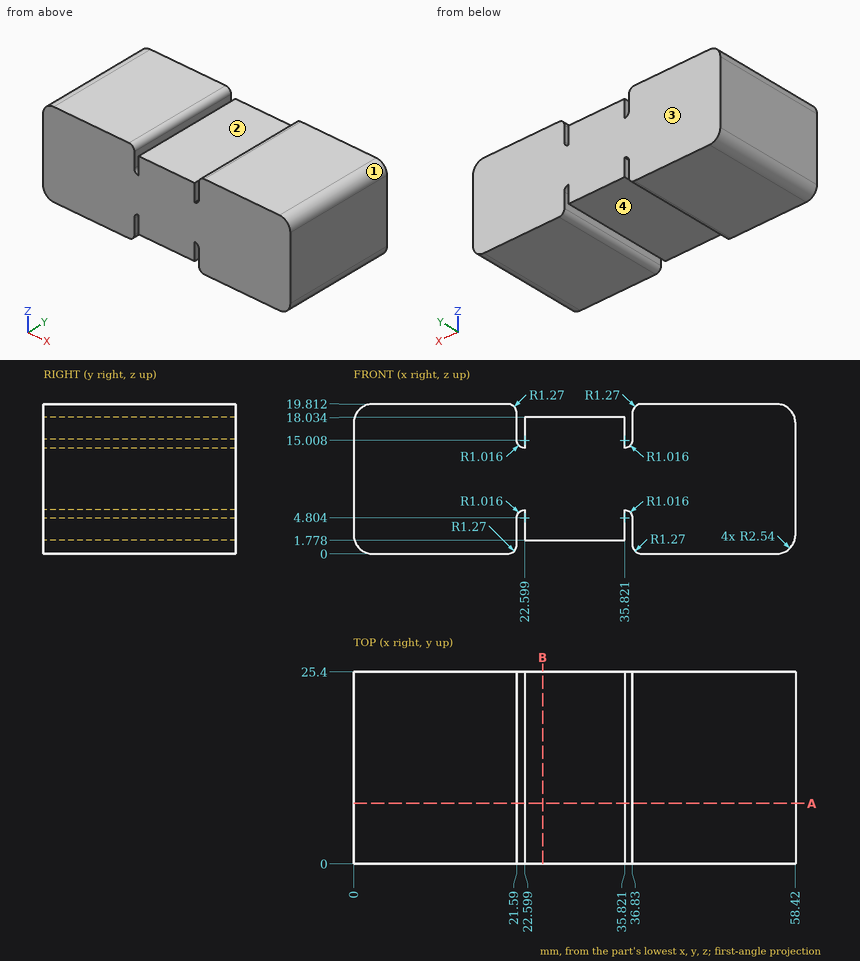
Here's the drawing with two shaded views (mm, measured from the low corner). I have some questions. Give positions to 0.01 mm unless a question says otherwise; leave off trailing zeros. Order: outer loops, then holes, each group sorted by start corner. A loop starts at its lowest first (then second) coordinate and runs counter-clockwise, first axis right, second up. Notation, with made-up numbers: (53, 61) -> (59, 61) arc R7 cw to (59, 74) -> close; hole circle Ø11 at (54, 53.25). An arc over 180 degrees is marked (long way). One line per item, written item: value. Start each with the question number.
1. I need wall thicknesses on probe 1 along X at (y, z) = (15, 2.75); probe 2 along X at (y, z) = (17.75, 5.25); probe 3 along Z at (x, y) = (25, 2). Which ranges of each line are inside material? Lowest first, please. Write a range as from..to.
2. Will these pins go through, and if not, where does the flat tip stop? pin 1 Ø4 at (x, y) = (29.5, 17) entering from +Z; pin 2 Ø6.5 at (x, y) = (31, 10.5) entering from -Z.
3. We'd pull the mould along X, two halves only. Please class the marked faces 1, 2, 3 and 4: released by +X, released by -X, zero draft, split by the parting line, or undercut.
4. Imagine slicing it at B-B, the plane x = 25. List the corners of the cut face in (y, z) for me, plus the area to 3 significant figures.
5. Imagine slicing it at A-A, the plane y = 8. List the corners of the cut face in (x, z) for me (1 decimal), plus the area to 3 significant figures.
Values follow:
1. probe 1: x = 0..21.59, 22.6..35.82, 36.83..58.42
1. probe 2: x = 0..21.69, 22.6..35.82, 36.73..58.42
1. probe 3: z = 1.78..18.03
2. pin 1: stops at z = 18.03
2. pin 2: stops at z = 1.78
3. face 1: released by +X
3. face 2: undercut
3. face 3: zero draft
3. face 4: undercut
4. outline: (0, 1.78) -> (25.4, 1.78) -> (25.4, 18.03) -> (0, 18.03) -> close
4. area: 413 mm2
5. outline: (0, 2.5) arc R2.5 ccw to (2.5, 0) -> (20.3, 0) arc R1.3 ccw to (21.6, 1.3) -> (21.6, 4.7) arc R1 cw to (22.6, 5.8) -> (22.6, 1.8) -> (35.8, 1.8) -> (35.8, 5.8) arc R1 cw to (36.8, 4.7) -> (36.8, 1.3) arc R1.3 ccw to (38.1, 0) -> (55.9, 0) arc R2.5 ccw to (58.4, 2.5) -> (58.4, 17.3) arc R2.5 ccw to (55.9, 19.8) -> (38.1, 19.8) arc R1.3 ccw to (36.8, 18.5) -> (36.8, 15.1) arc R1 cw to (35.8, 14) -> (35.8, 18) -> (22.6, 18) -> (22.6, 14) arc R1 cw to (21.6, 15.1) -> (21.6, 18.5) arc R1.3 ccw to (20.3, 19.8) -> (2.5, 19.8) arc R2.5 ccw to (0, 17.3) -> close
5. area: 1,080 mm2
